from build123d import *

# Parameters (mm, degrees)
FILLET1_R                       = 5.08
FILLET2_R                       = 1.27
BOSS_EXTRUDE1_REACH             = 19.048
SKETCH2_R                       = 4.7625
SKETCH2_W                       = 6.477
SKETCH2_H                       = 6.477
BOSS_EXTRUDE1_DIRECTION_2_REACH = 19.048
SKETCH3_W                       = 6.477
SKETCH3_H                       = 6.477
CUT_EXTRUDE1_DEPTH              = 18.047970635
SKETCH4_R                       = 5.207
CUT_EXTRUDE2_DEPTH              = 1.143
CHAMFER2_SIZE                   = 0.254


with BuildPart() as part:
    # Sketch1 → Revolve1 (revolve)
    with BuildSketch(Plane.XY, mode=Mode.PRIVATE) as revolve1_sk:
        Polygon((4.7625, 0), (4.7625, 3.302), (2.8575, 3.302), (2.8575, 9.398), (4.7625, 9.398), (4.7625, 12.7), (11.43, 12.7), (6.35, 6.35), (11.43, 0), align=None)
    revolve(revolve1_sk.sketch.rotate(Axis((0, 0, 0), (0, 1, 0)), 90), axis=Axis((0, 0, 0), (0, 1, 0)))

    # Fillet1
    fillet1_edges = [part.edges().sort_by_distance(p)[0] for p in [
        (0, 6.35, 6.35),
    ]]
    fillet(fillet1_edges, radius=FILLET1_R)

    # Fillet2
    fillet2_edges = [part.edges().sort_by_distance(p)[0] for p in [
        (0, 0, 11.43),
        (0, 12.7, 11.43),
    ]]
    fillet(fillet2_edges, radius=FILLET2_R)

    # Boss-Extrude1: up to this face of the body (flat: up to its plane)
    boss_extrude1_end = Plane(part.part.faces().sort_by_distance((0, 12.7, 8.539055399))[0])
    # Sketch2 → Boss-Extrude1 (add, up to the picked face)
    with BuildSketch(Plane(origin=(0, 9.398, 0), x_dir=(1, 0, 0), z_dir=(0, 1, 0)), mode=Mode.PRIVATE) as boss_extrude1_sk1:
        Circle(SKETCH2_R)
        Rectangle(SKETCH2_W, SKETCH2_H, mode=Mode.SUBTRACT)
    boss_extrude1_tool1 = split(extrude(boss_extrude1_sk1.sketch, amount=BOSS_EXTRUDE1_REACH, mode=Mode.PRIVATE), bisect_by=boss_extrude1_end, keep=Keep.BOTH, mode=Mode.PRIVATE)
    add(boss_extrude1_tool1.solids().sort_by(Axis((-4.627796, 9.398, 0), (0, 1, 0)))[0])

    # Boss-Extrude1 direction 2: up to this face of the body (flat: up to its plane)
    boss_extrude1_direction_2_end = Plane(part.part.faces().sort_by_distance((0, 0, 8.539055399))[0])
    # Sketch2 → Boss-Extrude1 direction 2 (add, up to the picked face)
    with BuildSketch(Plane(origin=(0, 9.398, 0), x_dir=(1, 0, 0), z_dir=(0, 1, 0)), mode=Mode.PRIVATE) as boss_extrude1_direction_2_sk1:
        Circle(SKETCH2_R)
        Rectangle(SKETCH2_W, SKETCH2_H, mode=Mode.SUBTRACT)
    boss_extrude1_direction_2_tool1 = split(extrude(boss_extrude1_direction_2_sk1.sketch, amount=-BOSS_EXTRUDE1_DIRECTION_2_REACH, mode=Mode.PRIVATE), bisect_by=boss_extrude1_direction_2_end, keep=Keep.BOTH, mode=Mode.PRIVATE)
    add(boss_extrude1_direction_2_tool1.solids().sort_by(Axis((-4.627796, 9.398, 0), (0, -1, 0)))[0])

    # Sketch3 → Cut-Extrude1 (cut, through all)
    with BuildSketch(Plane(origin=(0, 9.398, 0), x_dir=(1, 0, 0), z_dir=(0, 1, 0))):
        Rectangle(SKETCH3_W, SKETCH3_H)
    extrude(amount=-CUT_EXTRUDE1_DEPTH, mode=Mode.SUBTRACT)

    # Sketch4 → Cut-Extrude2 (cut)
    with BuildSketch(Plane(origin=(0, 12.7, 0), x_dir=(1, 0, 0), z_dir=(0, 1, 0))):
        with Locations(Location((0, 0, 0), (0, 0, 270))):
            Circle(SKETCH4_R)
    cut_extrude2 = extrude(amount=-CUT_EXTRUDE2_DEPTH, mode=Mode.SUBTRACT)

    # Mirror1: Cut-Extrude2 across plane
    add(cut_extrude2.mirror(Plane.ZX.offset(6.35)), mode=Mode.SUBTRACT)

    # Chamfer2
    chamfer2_edges = [part.edges().sort_by_distance(p)[0] for p in [
        (3.2385, 11.557, 0),
        (-3.2385, 11.557, 0),
        (0, 11.557, 3.2385),
        (0, 11.557, -3.2385),
        (0, 12.7, -5.207),
        (3.2385, 1.143, 0),
        (0, 0, -5.207),
        (0, 1.143, 3.2385),
        (-3.2385, 1.143, 0),
        (0, 1.143, -3.2385),
    ]]
    chamfer(chamfer2_edges, length=CHAMFER2_SIZE)


solid = part.part
The model under review builds one solid part; all positions refer to its coordinate system, in mm. A direction names the side the tool comes from. Give positions to 0.01 mm unless a question says otherwise; leave off trailing zeros. Answer as a JSON object with one key per item and string values. Group by question number.
Q1. Wall thickness on line 1 along Y through (x, z) = (-3.75, 1.75); line 2 along Y through (x, z) = (5, 8.25); line 3 along Y through (x, z) = (-9, -2): over which ranges is each line inside the solid? List them lowest first.
Q2. Insertion check: pin 1 (9.5 mm diameter, centred on x = 0, z = 0, fed in from -Y); pin 2 (3 mm diameter, centred on y = 4, z = -0.5, fed in from +X); pin 3 (3 mm diameter, centred on x = 7, y = 2, fed in from +Z). Each pin has a flat end and moves straight along its axis. Give the tip position at first contact, or say it passes through.
Q3. Tool access review of faces 1 (the flat face through (4, 12.7, 4)), 2 (the flat face through (0, 1.143, -4)), 3 (the cylindrical face through (1.564, 12.008, 4.967)), 4 (the flat face through (0, 6, -3.238)): name each direction out of +Z, -Z, +X, -X, +Y, -Y from which nothing blocks a thin tool from reaching the whole face with its end or side.
Q4. Draft analysis for pull direction Z (two halves, no side actions). For faces 5 (the flat face through (-4, 0, 4)), 6 (the flat face through (3.238, 6, 0)), 7 (the flat face through (-3.238, 6, 0)), state which applies: pulls with the +Z half, pulls with the -Z half, needs draft (parallel to the pull), parting line crosses it, or undercut.
Answer below:
{
 "1": {"line 1": "y = 1.14 to 11.56", "line 2": "y = 0.33 to 2.23, 10.47 to 12.37", "line 3": "y = 0.08 to 2.76, 9.94 to 12.62"},
 "2": {"pin 1": "stops at y = 1.14", "pin 2": "stops at x = 9.42", "pin 3": "stops at z = 8.34"},
 "3": {"face 1": "+Z, -Z, +X, -X, +Y", "face 2": "-Y", "face 3": "+Y", "face 4": "+Y, -Y"},
 "4": {"face 5": "needs draft", "face 6": "undercut", "face 7": "undercut"}
}
